The model under review builds one solid part; all positions refer to its coordinate system, in mm. Coordinates: 2 decimals unless noted, no trailing zeros. Write each loop counter-clockwise with the first axis right and the second up, starting at its lowest first coordinate (ties: lowest second). Pieces come first, ordered by that corner, then holes.
```python
from build123d import *

# Parameters (mm, degrees)
F0_W     = 1447.8
F0_H     = 406.4
F2_DEPTH = 12.7
F1_R     = 9.525
F1_R_2   = 6.35
F3_DEPTH = 355.6


with BuildPart() as f2:
    # F0 (on Top) → F2 (new body, symmetric)
    with BuildSketch(Plane.XY):
        Rectangle(F0_W, F0_H)
    extrude(amount=F2_DEPTH, both=True)

    # F1 (on Right) → F3 (join, symmetric)
    with BuildSketch(Plane.YZ):
        with Locations((-210.82, 0)):
            Circle(F1_R)
        with Locations((-210.82, 0)):
            Circle(F1_R_2, mode=Mode.SUBTRACT)
    extrude(amount=F3_DEPTH, both=True)


solid = f2.part
```
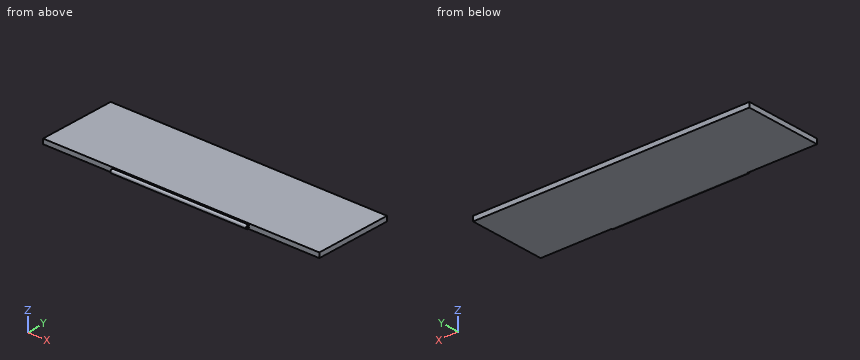
Item 1: For pin 1 (7.5 mm diameter, centred on x = -80.5, z = -6, fed in from -Y); pin 2 (8.5 mm diameter, centred on y = -212.5, z = 3.5, fed in from +X); pin 3 (7.5 mm diameter, centred on y = -210.82, z = 0, fed in from +X); pin 4 (1 mm diameter, centred on x = 19, z = -7.5, fed in from -Y), all flat-tipped, find the tip position at first contact; note any pin that passes through.
Solved:
pin 1: stops at y = -220.08
pin 2: stops at x = 355.6
pin 3: passes through
pin 4: stops at y = -217.28
Item 2: To check wall thickness, follow line 1 along Z through (x, y) = (-164, -210); line 2 along Y through (x, z) = (111, -7); line 3 along Y through (x, z) = (169, -0.75). State the ranges of each line that lie inside material, in increasing order.
Solved:
line 1: z = -9.49 to -6.3, 6.3 to 9.49
line 2: y = -217.28 to -204.36, -203.2 to 203.2
line 3: y = -220.32 to -217.13, -204.51 to 203.2
Item 3: Take a section at C-C, the plane x = -609. Write out the cut boundary in (y, z).
Solved:
outline: (-203.2, -12.7) - (203.2, -12.7) - (203.2, 12.7) - (-203.2, 12.7) - close
Item 4: Take a section at B-B, the plane x = -343. Write out the cut boundary in (y, z) (3 decimals).
Solved:
outline: (-203.2, -12.7) - (203.2, -12.7) - (203.2, 12.7) - (-203.2, 12.7) - (-203.2, 5.715) arc R9.525 ccw (long way) to (-203.2, -5.715) - close; hole circle Ø12.7 at (-210.82, 0)
Item 5: Take a section at A-A, the plane z = 0. Write out the cut boundary in (x, y) (3 decimals), plus the area to 3 significant figures.
Solved:
outline: (-723.9, -203.2) - (-355.6, -203.2) - (-355.6, -204.47) - (355.6, -204.47) - (355.6, -203.2) - (723.9, -203.2) - (723.9, 203.2) - (-723.9, 203.2) - close; (-355.6, -220.345) - (355.6, -220.345) - (355.6, -217.17) - (-355.6, -217.17) - close
area: 592,000 mm2
